Can you work these out from the model? Positions are in its coordinate system, mm. Face numbers are marked on the shaded views. A direction names the side the tool comes from. Round coordinates to 2 decimals unless told otherwise and drop trailing zeros. Order: outer loops, then holes, each group sorted by start corner. A loop starts at its lowest first (then second) coordinate and runs counter-clockwise, first axis right, second up. Notation, with made-up numbers: M 33.5,-20 L 77.5,-20 A27 ccw 77.5,8 Z; hole C 6,-27.75 d10. An arc over 180 degrees is marked long. One line per question, with ' | ' between items.
```python
from build123d import *

# Parameters (mm, degrees)
F0_W     = 64
F0_H     = 50
F1_DEPTH = 24
F3_DEPTH = 50


with BuildPart() as f1:
    # F0 (on Top) → F1 (new body)
    with BuildSketch(Plane.XY):
        with Locations((6, 0)):
            Rectangle(F0_W, F0_H)
    extrude(amount=F1_DEPTH)

    # F2 (on face) → F3 (cut)
    with BuildSketch(Plane.XZ.offset(25)):
        Polygon((30.3, 8), (30.3, 24), (-10.876341, 24), (-18, 8), align=None)
    extrude(amount=-F3_DEPTH, mode=Mode.SUBTRACT)


solid = f1.part
```
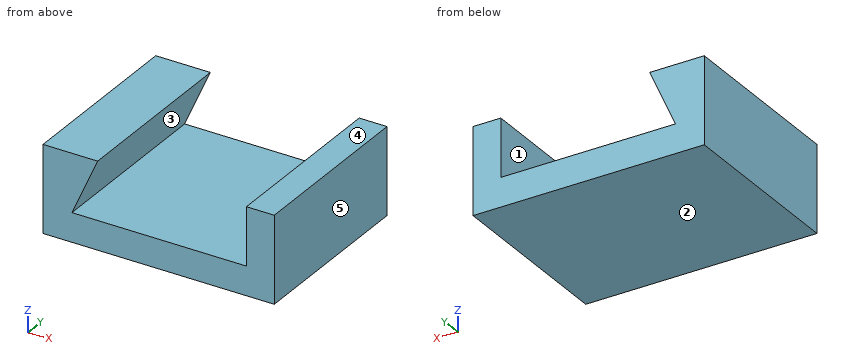
(1) If we section it at C-C on y = -14: Please give me the cut outline in (x, z), plus the area to 3 significant figures.
Final values:
outline: M -26,0 L 38,0 L 38,24 L 30.3,24 L 30.3,8 L -18,8 L -10.88,24 L -26,24 Z | area: 820 mm^2
(2) Please list where these lines run through material, in increasing order: probe 1 along Z at (x, y) = (11.5, 16); probe 2 along X at (y, z) = (11, 17); probe 3 along X at (y, z) = (23, 13.25). Write a range as [from, to].
Final values:
probe 1: [0, 8] | probe 2: [-26, -13.99], [30.3, 38] | probe 3: [-26, -15.66], [30.3, 38]
(3) If we section it at A-A on z = 22.75: Please give me the cut outline in (x, y), plus the area to 3 significant figures.
Final values:
outline: M -26,-25 L -11.43,-25 L -11.43,25 L -26,25 Z; M 30.3,-25 L 38,-25 L 38,25 L 30.3,25 Z | area: 1,110 mm^2
(4) Will this pin go through, and if not, where does the flat tip stop? pin 1 Ø14.5 at (x, y) = (2.5, -10) entering from +Z.
Final values:
pin 1: z = 8
(5) If we section it at D-D on x = 22: Please give me the cut outline in (y, z).
Final values:
outline: M -25,0 L 25,0 L 25,8 L -25,8 Z
(6) On a 3-axis mill with a long thin cutter (end or side, diameter ignored), from which of +Z, -Z, +X, -X, +Y, -Y can I reach the whole of each face in a straight line? I mean the marked faces 1 and 2. Say none if no direction works.
Final values:
face 1: +Z, +Y, -Y | face 2: -Z, +X, -X, +Y, -Y
(7) Thinking about a two-plate mould opening in X: for the marked faces 3, 4 and 5, which applies, released by +X, released by -X, zero draft, split by the parting line, or undercut?
Final values:
face 3: undercut | face 4: zero draft | face 5: released by +X
(8) If we section it at B-B on x = -17: Please give me the cut outline in (y, z), plus the area to 3 significant figures.
Final values:
outline: M -25,0 L 25,0 L 25,8 L -25,8 Z; M -25,10.25 L 25,10.25 L 25,24 L -25,24 Z | area: 1,090 mm^2
